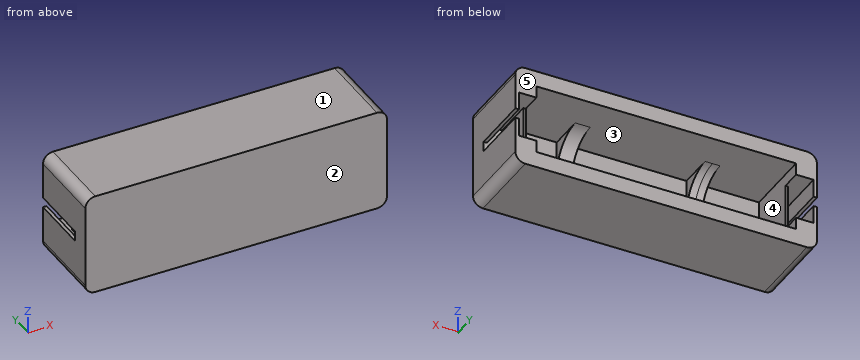
from build123d import *

# Parameters (mm, degrees)
SKETCH2_W                                  = 60.4
SKETCH2_H                                  = 20.4
BOSS_EXTRUDE1_DEPTH                        = 16
SKETCH3_W                                  = 52
SKETCH3_H                                  = 14
CUT_EXTRUDE1_DEPTH                         = 14
FILLET1_R                                  = 2
SKETCH4_W                                  = 0.5
SKETCH4_H                                  = 4.6
CUT_EXTRUDE2_DEPTH                         = 4
SKETCH5_W                                  = 3
SKETCH5_H                                  = 4.6
CUT_EXTRUDE3_DEPTH                         = 12
MIRROR5_COPY_1_SKETCH_W                    = 0.5
MIRROR5_COPY_1_SKETCH_H                    = 4.6
MIRROR5_COPY_1_DEPTH                       = 4
MIRROR5_COPY_2_SKETCH_W                    = 3
MIRROR5_COPY_2_SKETCH_H                    = 4.6
MIRROR5_COPY_2_DEPTH                       = 12
MIRROR5_COPY_3_SKETCH_W                    = 0.5
MIRROR5_COPY_3_SKETCH_H                    = 4.6
MIRROR5_COPY_3_DEPTH                       = 4
SKETCH8_W                                  = 3
SKETCH8_H                                  = 14
BOSS_EXTRUDE2_DEPTH                        = 7
CUT_EXTRUDE5_REACH                         = 49.183
SKETCH7_R                                  = 7
CUT_EXTRUDE5_DIRECTION_2_REACH             = 49.183
SKETCH9_W                                  = 0.7
SKETCH9_H                                  = 1
CUT_EXTRUDE6_DEPTH                         = 12
MIRROR8_AT_THE_SECOND_PLANE_COPY_1_SKETC_W = 0.7
MIRROR8_AT_THE_SECOND_PLANE_COPY_1_SKETC_H = 1
MIRROR8_AT_THE_SECOND_PLANE_COPY_1_DEPTH   = 12


with BuildPart() as part:
    # Sketch2 → Boss-Extrude1 (new body)
    with BuildSketch(Plane(origin=(0, 0, 0), x_dir=(1, 0, 0), z_dir=(0, 1, 0))):
        Rectangle(SKETCH2_W, SKETCH2_H)
    extrude(amount=BOSS_EXTRUDE1_DEPTH)

    # Sketch3 → Cut-Extrude1 (cut)
    with BuildSketch(Plane(origin=(0, 16, 0), x_dir=(1, 0, 0), z_dir=(0, 1, 0))):
        Rectangle(SKETCH3_W, SKETCH3_H)
    extrude(amount=-CUT_EXTRUDE1_DEPTH, mode=Mode.SUBTRACT)

    # Fillet1
    fillet1_edges = [part.edges().sort_by_distance(p)[0] for p in [
        (30.2, 8, 10.2),
        (-30.2, 8, 10.2),
        (-30.2, 8, -10.2),
        (30.2, 8, -10.2),
    ]]
    fillet(fillet1_edges, radius=FILLET1_R)

    # Sketch4 → Cut-Extrude2 (cut)
    with BuildSketch(Plane(origin=(0, 16, 0), x_dir=(1, 0, 0), z_dir=(0, 1, 0))):
        with Locations((-26.25, 2.3)):
            Rectangle(SKETCH4_W, SKETCH4_H)
    cut_extrude2 = extrude(amount=-CUT_EXTRUDE2_DEPTH, mode=Mode.SUBTRACT)

    # Sketch5 → Cut-Extrude3 (cut)
    with BuildSketch(Plane(origin=(0, 16, 0), x_dir=(1, 0, 0), z_dir=(0, 1, 0))):
        with Locations((-28, 2.3)):
            Rectangle(SKETCH5_W, SKETCH5_H)
    cut_extrude3 = extrude(amount=-CUT_EXTRUDE3_DEPTH, mode=Mode.SUBTRACT)

    # Mirror4: Cut-Extrude2, Cut-Extrude3 across plane
    add(cut_extrude2.mirror(Plane(origin=(0, 0, 0), x_dir=(0, 0, 1), z_dir=(1, 0, 0))), mode=Mode.SUBTRACT)
    add(cut_extrude3.mirror(Plane(origin=(0, 0, 0), x_dir=(0, 0, 1), z_dir=(1, 0, 0))), mode=Mode.SUBTRACT)

    # Mirror5: Cut-Extrude3 across plane
    add(cut_extrude3.mirror(Plane.XY), mode=Mode.SUBTRACT)

    # Mirror5 copy 1 sketch → Mirror5 copy 1 (cut)
    with BuildSketch(Plane(origin=(0, 16, 0), x_dir=(-1, 0, 0), z_dir=(0, 1, 0))):
        with Locations((-26.25, 2.3)):
            Rectangle(MIRROR5_COPY_1_SKETCH_W, MIRROR5_COPY_1_SKETCH_H)
    extrude(amount=-MIRROR5_COPY_1_DEPTH, mode=Mode.SUBTRACT)

    # Mirror5 copy 2 sketch → Mirror5 copy 2 (cut)
    with BuildSketch(Plane(origin=(0, 16, 0), x_dir=(-1, 0, 0), z_dir=(0, 1, 0))):
        with Locations((-28, 2.3)):
            Rectangle(MIRROR5_COPY_2_SKETCH_W, MIRROR5_COPY_2_SKETCH_H)
    extrude(amount=-MIRROR5_COPY_2_DEPTH, mode=Mode.SUBTRACT)

    # Mirror5 copy 3 sketch → Mirror5 copy 3 (cut)
    with BuildSketch(Plane(origin=(0, 16, 0), x_dir=(1, 0, 0), z_dir=(0, 1, 0))):
        with Locations((-26.25, -2.3)):
            Rectangle(MIRROR5_COPY_3_SKETCH_W, MIRROR5_COPY_3_SKETCH_H)
    extrude(amount=-MIRROR5_COPY_3_DEPTH, mode=Mode.SUBTRACT)

    # Sketch8 → Boss-Extrude2 (add)
    with BuildSketch(Plane(origin=(0, 2, 0), x_dir=(1, 0, 0), z_dir=(0, 1, 0))):
        with Locations((-13, 0)):
            Rectangle(SKETCH8_W, SKETCH8_H)
    boss_extrude2 = extrude(amount=BOSS_EXTRUDE2_DEPTH)

    # Sketch7 → Cut-Extrude5 (cut, up to next)
    with BuildSketch(Plane(origin=(-13, 0, 0), x_dir=(0, 0, -1), z_dir=(1, 0, 0)), mode=Mode.PRIVATE) as cut_extrude5_sk1:
        with Locations((0, 9)):
            Circle(SKETCH7_R)
    cut_extrude5_tool1 = extrude(cut_extrude5_sk1.sketch, amount=-CUT_EXTRUDE5_REACH, mode=Mode.PRIVATE) & part.part
    cut_extrude5 = cut_extrude5_tool1.solids().sort_by_distance((-13, 9, 0))[0]
    add(cut_extrude5, mode=Mode.SUBTRACT)

    # Sketch7 → Cut-Extrude5 direction 2 (cut, up to next)
    with BuildSketch(Plane(origin=(-13, 0, 0), x_dir=(0, 0, -1), z_dir=(1, 0, 0)), mode=Mode.PRIVATE) as cut_extrude5_direction_2_sk1:
        with Locations((0, 9)):
            Circle(SKETCH7_R)
    cut_extrude5_direction_2_tool1 = extrude(cut_extrude5_direction_2_sk1.sketch, amount=CUT_EXTRUDE5_DIRECTION_2_REACH, mode=Mode.PRIVATE) & part.part
    cut_extrude5_direction_2 = cut_extrude5_direction_2_tool1.solids().sort_by_distance((-13, 9, 0))[0]
    add(cut_extrude5_direction_2, mode=Mode.SUBTRACT)

    # Mirror7: Boss-Extrude2, Cut-Extrude5, Cut-Extrude5 direction 2 across plane
    add(boss_extrude2.mirror(Plane(origin=(0, 0, 0), x_dir=(0, 0, 1), z_dir=(1, 0, 0))))
    add(cut_extrude5.mirror(Plane(origin=(0, 0, 0), x_dir=(0, 0, 1), z_dir=(1, 0, 0))), mode=Mode.SUBTRACT)
    add(cut_extrude5_direction_2.mirror(Plane(origin=(0, 0, 0), x_dir=(0, 0, 1), z_dir=(1, 0, 0))), mode=Mode.SUBTRACT)

    # Sketch9 → Cut-Extrude6 (cut)
    with BuildSketch(Plane(origin=(0, 16, 0), x_dir=(1, 0, 0), z_dir=(0, 1, 0))):
        with Locations((-29.85, 0.5)):
            Rectangle(SKETCH9_W, SKETCH9_H)
    cut_extrude6 = extrude(amount=-CUT_EXTRUDE6_DEPTH, mode=Mode.SUBTRACT)

    # Mirror8: Cut-Extrude6 across plane
    add(cut_extrude6.mirror(Plane.XY), mode=Mode.SUBTRACT)

    # Mirror8 at the second plane: Cut-Extrude6 across plane
    add(cut_extrude6.mirror(Plane(origin=(0, 0, 0), x_dir=(0, 0, 1), z_dir=(1, 0, 0))), mode=Mode.SUBTRACT)

    # Mirror8 at the second plane copy 1 sketc → Mirror8 at the second plane copy 1 (cut)
    with BuildSketch(Plane(origin=(0, 16, 0), x_dir=(-1, 0, 0), z_dir=(0, 1, 0))):
        with Locations((-29.85, 0.5)):
            Rectangle(MIRROR8_AT_THE_SECOND_PLANE_COPY_1_SKETC_W, MIRROR8_AT_THE_SECOND_PLANE_COPY_1_SKETC_H)
    extrude(amount=-MIRROR8_AT_THE_SECOND_PLANE_COPY_1_DEPTH, mode=Mode.SUBTRACT)


solid = part.part
The listing builds one solid part. Answer for the finished solid, in the listing's coordinates (mm). Face numbers are marked on the shaded views. A direction names the side the tool comes from. Coordinates: 2 decimals unless noted, no trailing zeros. Write each loop counter-clockwise with the first axis right and the second up, starting at its lowest first coordinate (ties: lowest second). Pieces come first, ordered by that corner, then holes. Notation, with made-up numbers: M 11,35 L 50,35 A7 ccw 50,46 Z; hole C 50.5,84.25 d10. An arc over 180 degrees is marked long. Write each question's results on one line, items separated by ' | '.
Item 1: For a pull along Z with two mould halves and no side action, classify the marked faces 1, 2 and 3 as released by +Z, released by -Z, zero draft, split by the parting line, or undercut.
Answer below:
face 1: released by +Z | face 2: zero draft | face 3: undercut
Item 2: Which of the six approach directions +Z, -Z, +X, -X, +Y, -Y give full straight-line access (tool end or side, diameter ignored) to the marked faces 4 and 5?
Answer below:
face 4: +Y | face 5: +Z, -Z, +X, -X, +Y
Item 3: Consider probe 1 along X at (y, z) = (9, 2.25); probe 2 along Z at (x, y) = (4, 7.5); probe 3 along X at (y, z) = (12.75, 3.75). Determine where each line is inside the solid, lowest interval first. Write a range as [from, to].
Answer below:
probe 1: [-30.2, -29.5], [-26.5, -26], [26, 26.5], [29.5, 30.2] | probe 2: [-10.2, -7], [7, 10.2] | probe 3: [-30.2, -29.5], [29.5, 30.2]
Item 4: The part is cut by section B-B on y = 15.25. Determine the outline of the cut face in (x, z).
Answer below:
outline: M -30.2,-8.2 A2 ccw -28.2,-10.2 L 28.2,-10.2 A2 ccw 30.2,-8.2 L 30.2,-1 L 29.5,-1 L 29.5,-4.6 L 26,-4.6 L 26,-7 L -26,-7 L -26,-4.6 L -29.5,-4.6 L -29.5,-1 L -30.2,-1 Z; M -30.2,1 L -29.5,1 L -29.5,4.6 L -26,4.6 L -26,7 L 26,7 L 26,4.6 L 29.5,4.6 L 29.5,1 L 30.2,1 L 30.2,8.2 A2 ccw 28.2,10.2 L -28.2,10.2 A2 ccw -30.2,8.2 Z
Item 5: The part is cut by section C-C on x = 12.5. Determine the outline of the cut face in (y, z).
Answer below:
outline: M 0,-10.2 L 16,-10.2 L 16,-7 L 9,-7 A7 cw 9,7 L 16,7 L 16,10.2 L 0,10.2 Z
Item 6: The part is cut by section D-D on z = -3.5. Determine the outline of the cut face in (x, y).
Answer below:
outline: M -30.2,0 L 30.2,0 L 30.2,16 L 29.5,16 L 29.5,4 L 26.5,4 L 26.5,12 L 26,12 L 26,2 L 14.5,2 L 14.5,2.94 L 11.5,2.94 L 11.5,2 L -11.5,2 L -11.5,2.94 L -14.5,2.94 L -14.5,2 L -26,2 L -26,12 L -26.5,12 L -26.5,4 L -29.5,4 L -29.5,16 L -30.2,16 Z
Item 7: Given P1, Ø1.9, axis at x = 28.5, z = 2.5, coming from the +Y side; P2, Ø6, axis at x = 19, z = -2, coming from the +Y side, each flat-ended and moving along its own axis, determine where each tip first touches the part or whether it passes through.
Answer below:
P1: y = 4 | P2: y = 2
Item 8: The part is cut by section A-A on y = 11.25. Determine the outline of the cut face in (x, z).
Answer below:
outline: M -30.2,-8.2 A2 ccw -28.2,-10.2 L 28.2,-10.2 A2 ccw 30.2,-8.2 L 30.2,-1 L 29.5,-1 L 29.5,-4.6 L 26.5,-4.6 L 26.5,4.6 L 29.5,4.6 L 29.5,1 L 30.2,1 L 30.2,8.2 A2 ccw 28.2,10.2 L -28.2,10.2 A2 ccw -30.2,8.2 L -30.2,1 L -29.5,1 L -29.5,4.6 L -26.5,4.6 L -26.5,-4.6 L -29.5,-4.6 L -29.5,-1 L -30.2,-1 Z; hole M -26,-7 L 26,-7 L 26,7 L -26,7 Z
